Work out the finished part from the listing and answer in its coordinate system (mm). Face numbers are marked on the shaded views. A direction names the side the tool comes from. Coordinates: 2 decimals unless noted, no trailing zeros. Order: outer loops, then holes, each group sorted by start corner. A loop starts at its lowest first (then second) coordinate and runs counter-clockwise, first axis right, second up.
1. A tool of negligible diameter and unlimited length cuts with its end or side. For the marked faces 1, 2, 3, 4 and 5, from which of +Z, -Z, +X, -X, +Y, -Y can it reach the whole face along a straight path? Write none if from no direction.
2. The part is cut by section B-B, the plane y = -16. Give the vertices of the cut face in (x, z).
3. Flat-ended cylindrical pins translate along their axes: pin 1 Ø4 at (y, z) = (-12, 48.5) entering from +X; pin 2 Ø5 at (x, y) = (-49.5, -18.5) entering from +Z; pin 3 Ø8 at (x, y) = (0, -10) entering from +Z; pin 4 Ø9.5 at (x, z) = (-152.4, 0) entering from -Y. Find the tip coordinate at first contact, or state that the pin passes through.
4. Find the intervals of material crossed by probe 1 along Z at (x, y) = (-152.4, -15.5); probe 2 along X at (y, z) = (-7.5, 4); probe 3 along X at (y, z) = (-17.25, -4.5), in increasing order.
5. The part is cut by section C-C, the plane x = -70.5. Give the vertices of the cut face in (y, z).
6. The part is cut by section A-A, the plane z = 0. Give the vertices of the cut face in (x, y).
7. Determine the mould class of the marked faces 6, 7 and 8 for opening direction Z: +Z half, -Z half, draft (parallel to the pull), parting line (faces both ways), or undercut.
8. The part is cut by section D-D, the plane z = 46. Give the vertices of the cut face in (x, y), then the cut area to 3 significant figures.
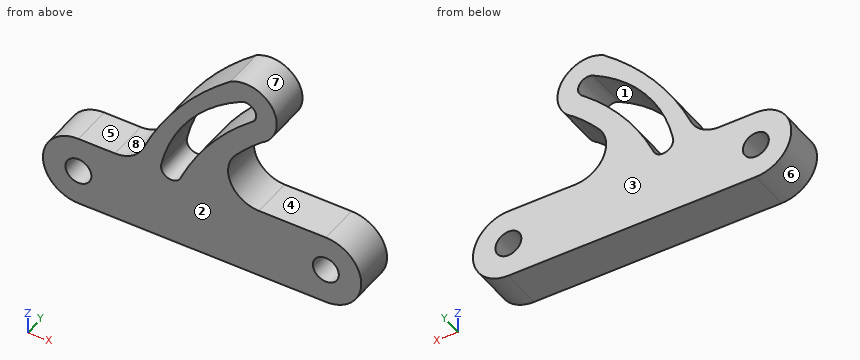
```python
from build123d import *

# Parameters (mm, degrees)
F0_R     = 8.001
F1_DEPTH = 25.4


with BuildPart() as f1:
    # F0 (on Front) → F1 (new body)
    with BuildSketch(Plane.XZ):
        with BuildLine():
            Line((-76.2, -21.844), (0, -21.844))
            ThreePointArc((0, -21.844), (21.844, 0), (0, 21.844))
            Line((0, 21.844), (-41.175205, 21.844))
            ThreePointArc((-41.175205, 21.844), (-58.513323, 33.001463), (-55.541791, 53.404144))
            ThreePointArc((-55.541791, 53.404144), (-47.955418, 61.443356), (-39.751, 68.850752))
            ThreePointArc((-39.751, 68.850752), (-32.778216, 94.873536), (-58.801, 101.84632))
            ThreePointArc((-58.801, 101.84632), (-89.907606, 70.913561), (-112.392814, 33.245646))
            ThreePointArc((-112.392814, 33.245646), (-119.418861, 24.947156), (-129.840026, 21.844))
            Line((-129.840026, 21.844), (-152.4, 21.844))
            ThreePointArc((-152.4, 21.844), (-174.244, 0), (-152.4, -21.844))
            Line((-152.4, -21.844), (-76.2, -21.844))
        make_face()
        with Locations((-152.4, 0)):
            Circle(F0_R, mode=Mode.SUBTRACT)
        Circle(F0_R, mode=Mode.SUBTRACT)
        with BuildLine():
            ThreePointArc((-52.451, 90.847797), (-43.776739, 88.523536), (-46.101, 79.849274))
            ThreePointArc((-46.101, 79.849274), (-70.902285, 54.405237), (-89.060293, 23.863634))
            ThreePointArc((-89.060293, 23.863634), (-96.837423, 19.373506), (-101.327551, 27.150635))
            ThreePointArc((-101.327551, 27.150635), (-84.079326, 64.516336), (-52.451, 90.847797))
        make_face(mode=Mode.SUBTRACT)
    extrude(amount=F1_DEPTH)


solid = f1.part
```
Geometry says:
1. face 1: +Y, -Y
1. face 2: +Z, -Z, +X, -X, -Y
1. face 3: +Z, -Z, +X, -X, +Y
1. face 4: +X, +Y, -Y
1. face 5: +Z, -X, +Y, -Y
2. outline: (-152.4, -21.84) - (0, -21.84) arc R21.84 ccw to (0, 21.84) - (-41.18, 21.84) arc R19.05 cw to (-55.54, 53.4) arc R138.24 cw to (-39.75, 68.85) arc R19.05 ccw to (-58.8, 101.85) arc R175.9 ccw to (-112.39, 33.25) arc R19.05 cw to (-129.84, 21.84) - (-152.4, 21.84) arc R21.84 ccw to start; hole circle Ø16 at (-152.4, 0); hole (-101.33, 27.15) arc R6.35 ccw to (-89.06, 23.86) arc R150.77 cw to (-46.1, 79.85) arc R6.35 ccw to (-52.45, 90.85) arc R93.44 ccw to start; hole circle Ø16 at (0, 0)
3. pin 1: stops at x = -57.63
3. pin 2: stops at z = 104.4
3. pin 3: stops at z = 21.84
3. pin 4: passes through
4. probe 1: z = -21.84 to -8, 8 to 21.84
4. probe 2: x = -173.87 to -159.33, -145.47 to -6.93, 6.93 to 21.47
4. probe 3: x = -173.78 to -159.02, -145.78 to -6.62, 6.62 to 21.38
5. outline: (-25.4, -21.84) - (0, -21.84) - (0, 54.93) - (-25.4, 54.93) - close; (-25.4, 78.8) - (0, 78.8) - (0, 91.97) - (-25.4, 91.97) - close
6. outline: (-174.24, -25.4) - (-160.4, -25.4) - (-160.4, 0) - (-174.24, 0) - close; (-144.4, -25.4) - (-8, -25.4) - (-8, 0) - (-144.4, 0) - close; (8, -25.4) - (21.84, -25.4) - (21.84, 0) - (8, 0) - close
7. face 6: parting line
7. face 7: undercut
7. face 8: +Z half
8. outline: (-106.18, -25.4) - (-95.15, -25.4) - (-95.15, 0) - (-106.18, 0) - close; (-76.91, -25.4) - (-59.53, -25.4) - (-59.53, 0) - (-76.91, 0) - close
8. area: 722 mm2
